Geometry check sheet. Reference: the model listing, model coordinates, mm. Face numbers are marked on the shaded views. A direction names the side the tool comes from. Give positions to 0.01 mm unless a question says otherwise; leave off trailing zeros. Order: outer loops, then holes, each group sorted by start corner. A loop starts at its lowest first (then second) coordinate and runs counter-clockwise, first axis right, second up. Notation, with made-up numbers: M 50.5,51 L 77.5,51 A21 cw 77.5,84 Z; hole C -35.5,4.5 d7. An arc over 180 degrees is marked long. Answer as CSV lines item,"result".
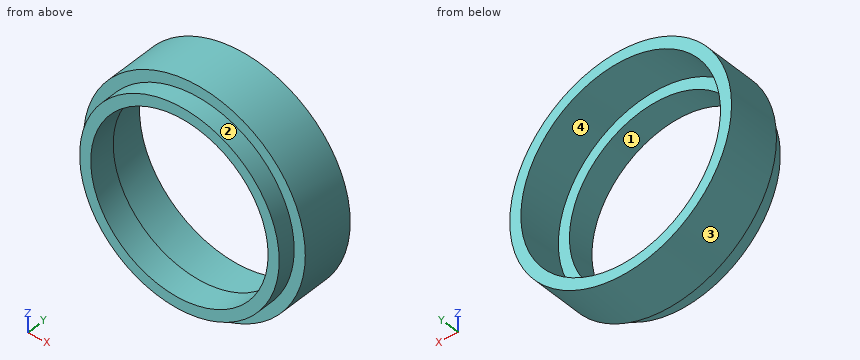
Autodesk Inventor part; units mm, degrees
ref_plane "YZ Plane" through (0, 0, 0) normal (1, 0, 0) x (0, 1, 0)
ref_plane "XZ Plane" through (0, 0, 0) normal (0, 1, 0) x (-1, 0, 0)
ref_plane "XY Plane" through (0, 0, 0) normal (0, 0, 1) x (1, 0, 0)
sketch "Sketch1" plane through (0, 0, 0) normal (0, 0, 1) x (1, 0, 0)
  line L0 (14.2875, 0) -> (14.2875, 2.54)
  line L1 (14.2875, 2.54) -> (15.875, 2.54)
  line L2 (15.875, 2.54) -> (15.875, 10.16)
  line L3 (15.875, 10.16) -> (0, 10.16)
  line L4 (14.2875, 0) -> (0, 0)
  line L5 (0, 10.16) -> (0, 0)
  dimension "d0" = 14.2875
  dimension "d1" = 15.875
  dimension "d2" = 2.54
  dimension "d3" = 7.62
revolve "Revolution1" add sketch "Sketch1" angle 360 about axis through (0, 10.16, 0) along (0, -1, 0)
thread "Thread1"
sketch "Sketch3" plane through (0, 10.16, 0) normal (0, 1, 0) x (1, 0, 0)
  circle A0 centre (0, 0) radius 14.2875
  dimension "d7" = 28.575
extrude "Extrusion1" cut sketch "Sketch3" against normal blind 6.35
sketch "Sketch4" plane through (0, 0, 0) normal (0, -1, 0) x (1, 0, 0)
  circle A0 centre (0, 0) radius 12.7
  dimension "d10" = 25.4
extrude "Extrusion2" cut sketch "Sketch4" against normal up to next
thread "Thread2"
properties part number "simulatedFilter" material "PET Plastic"
(1) Gauge pin test, flat ends, axial feed: P1, Ø2, axis at x = -12, y = 3.5, coming from the -Z side; P2, Ø6, axis at y = 5.5, z = 10, coming from the -X side; P3, Ø1.5, axis at x = -12.5, y = 4, coming from the -Z side. Record the tip position at first contact, or that the pin passes through.
The answers:
P1,"stops at z = -11.45"
P2,"stops at x = -14.25"
P3,"stops at z = -10.67"
(2) Section check B-B on x = 0. Enter the section's corners in (y, z) (1 decimal), then the cut area to 3 significant figures.
The answers:
outline,"M 0,-14.3 L 2.5,-14.3 L 2.5,-15.9 L 10.2,-15.9 L 10.2,-14.3 L 3.8,-14.3 L 3.8,-12.7 L 0,-12.7 Z; M 0,12.7 L 3.8,12.7 L 3.8,14.3 L 10.2,14.3 L 10.2,15.9 L 2.5,15.9 L 2.5,14.3 L 0,14.3 Z"
area,"36.3 mm2"
(3) Tool access check on the marked faces 3 and 4. Record the directions out of +Z, -Z, +X, -X, +Y, -Y that give a thin tool (end or side, any length) a straight path to the whole face; none if there is none.
The answers:
face 3,"+Y, -Y"
face 4,"+Y"
(4) Section check D-D on y = 1.25. Enter the section's corners in (x, z) (1 decimal), then the cut area to 3 significant figures.
The answers:
outline,"C 0,0 d28.6; hole C 0,0 d25.4"
area,"135 mm2"
(5) Section check A-A on z = 0. Enter the section's corners in (x, y) (1 decimal), then the cut area to 3 significant figures.
The answers:
outline,"M -15.9,2.5 L -14.3,2.5 L -14.3,0 L -12.7,0 L -12.7,3.8 L -14.3,3.8 L -14.3,10.2 L -15.9,10.2 Z; M 12.7,0 L 14.3,0 L 14.3,2.5 L 15.9,2.5 L 15.9,10.2 L 14.3,10.2 L 14.3,3.8 L 12.7,3.8 Z"
area,"36.3 mm2"
(6) Draft check along Z on the marked faces 1 and 2. Enter one of: +Z half, -Z half, draft (parallel to the pull), parting line (faces both ways), or undercut.
The answers:
face 1,"undercut"
face 2,"parting line"
(7) Material ranges on line 1 (Z direction, x = 0, y = 6.75) (1 decimal); line 2 (X direction, y = 9.75, z = -0.5); line 3 (X direction, y = 4.25, z = -4.5), recorded low to high.
The answers:
line 1,"z = -15.9 to -14.3, 14.3 to 15.9"
line 2,"x = -15.87 to -14.28, 14.28 to 15.87"
line 3,"x = -15.22 to -13.56, 13.56 to 15.22"
